The listing builds one solid part. Answer for the finished solid, in the listing's coordinates (mm). Round coordinates to 2 decimals unless told otherwise and drop trailing zeros. Write each loop counter-clockwise with the first axis right and the second up, starting at its lowest first coordinate (ties: lowest second). Pieces come first, ordered by that corner, then holes.
from build123d import *

# Parameters (mm, degrees)
F0_W      = 306.0099184513
F0_H      = 128.4345835447
F1_DEPTH  = 977.9
F3_DEPTH  = 508
F5_DEPTH  = 1577.34
F6_W      = 96.3038355112
F6_H      = 26.3143703341
F7_DEPTH  = 2032
F9_DEPTH  = 2032
F11_DEPTH = 2032


with BuildPart() as f1:
    # F0 (on Front) → F1 (new body)
    with BuildSketch(Plane.XZ):
        with Locations((-153.0049592257, 64.2172917724)):
            Rectangle(F0_W, F0_H)
    extrude(amount=F1_DEPTH)

    # F2 (on face) → F3 (cut)
    with BuildSketch(Plane.YZ):
        Polygon((-625.8537769318, 0), (-977.9, 102.1202132106), (-977.9, 0), align=None)
        Polygon((-352.044, 0), (0, 0), (0, 102.1202132106), align=None)
    extrude(amount=-F3_DEPTH, mode=Mode.SUBTRACT)

    # F4 (on face) → F5 (cut)
    with BuildSketch(Plane.XZ.offset(977.9)):
        Polygon((-136.761367321, 0), (-306.0099184513, 102.1202132106), (-306.0099184513, 0), align=None)
    extrude(amount=-F5_DEPTH, mode=Mode.SUBTRACT)

    # F6 (on face) → F7 (cut)
    with BuildSketch(Plane(origin=(0, 0, 0), x_dir=(-1, 0, 0), z_dir=(0, 1, 0))):
        with Locations((257.8580006957, 115.2773983777)):
            Rectangle(F6_W, F6_H)
    extrude(amount=-F7_DEPTH, mode=Mode.SUBTRACT)

    # F8 (on face) → F9 (cut)
    with BuildSketch(Plane.XY.offset(128.4345835447)):
        Polygon((-223.3109489244, -475.2492566424), (-104.8530414701, 0), (-310.773730278, 0), (-310.773730278, -104.1196882725), align=None)
        Polygon((-104.8530414701, -977.9), (-223.3109489244, -475.2492566424), (-310.773730278, -826.1470794678), (-310.773730278, -977.9), align=None)
        Polygon((-310.773730278, -826.1470794678), (-223.3109489244, -475.2492566424), (-310.773730278, -104.1196882725), align=None)
    extrude(amount=-F9_DEPTH, mode=Mode.SUBTRACT)

    # F10 (on face) → F11 (cut)
    with BuildSketch(Plane.XY.offset(128.4345835447)):
        Polygon((-184.1263636062, -641.520646722), (-174.1903899803, -278.1791781165), (-476.8389761448, -662.8549098969), align=None)
    extrude(amount=-F11_DEPTH, mode=Mode.SUBTRACT)


solid = f1.part
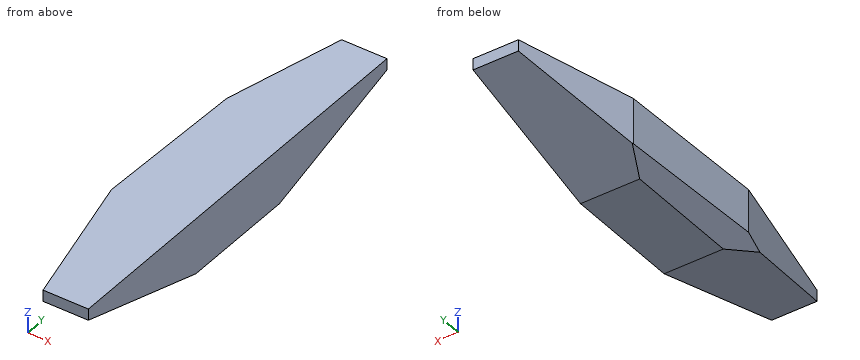
1. Section B-B on x = -33 is taken. Determine the outline of the cut face in (y, z).
Geometry says:
outline: (-977.9, 102.12) - (-625.85, 0) - (-352.04, 0) - (0, 102.12) - (0, 128.43) - (-977.9, 128.43) - close
2. Straight lines are drawn through the part: line 1 along X through (y, z) = (-496, 9.5); line 2 along X through (y, z) = (-514.5, 105); line 3 along Z through (x, y) = (-39, -102.5). For each, find the intervals that lie inside material, in ascending order.
Geometry says:
line 1: x = -152.51 to 0
line 2: x = -180.65 to 0
line 3: z = 72.39 to 128.43
3. Section C-C on y = -453.5 is taken. Determine the outline of the cut face in (x, z), plus the area to 4 significant figures.
Geometry says:
outline: (-178.98, 25.48) - (-136.76, 0) - (0, 0) - (0, 128.43) - (-178.98, 128.43) - close
area: 22,450 mm2
4. Given pin 1 (1.5 mm diameter, centred on y = -661, z = 20.5, fed in from -X); pin 2 (1.5 mm diameter, centred on x = -84, y = -243.5, fed in from -Z), each flat-ended and moving along its own axis, determine where each tip first touches the part or whether it passes through.
Geometry says:
pin 1: stops at x = -171.98
pin 2: stops at z = 31.27
5. Section D-D on y = -553.5 is taken. Determine the outline of the cut face in (x, z).
Geometry says:
outline: (-181.72, 27.13) - (-136.76, 0) - (0, 0) - (0, 128.43) - (-181.72, 128.43) - close
6. Section A-A on z = 118 is taken. Determine the outline of the cut face in (x, y).
Geometry says:
outline: (-184.13, -641.52) - (-104.85, -977.9) - (0, -977.9) - (0, 0) - (-104.85, 0) - (-174.19, -278.18) - close
